Geometry check sheet. Reference: drawing and pictorial views, mm from the part's lowest x, y, z. Round coordinates to 2 decimals unless told otherwise and drop trailing zeros. Loops run counter-clockwise (first coordinate to the right, second up) from the corner with the lowest first, then second, coordinate; pieces in that order, holes last. Notation, with made-up numbers: (80, 78.25) -> (114, 78.25) arc R35 ccw to (114, 111.25) -> close; hole circle Ø9 at (78, 60). An arc over 180 degrees is marked (long way). Write item = value, one per line.
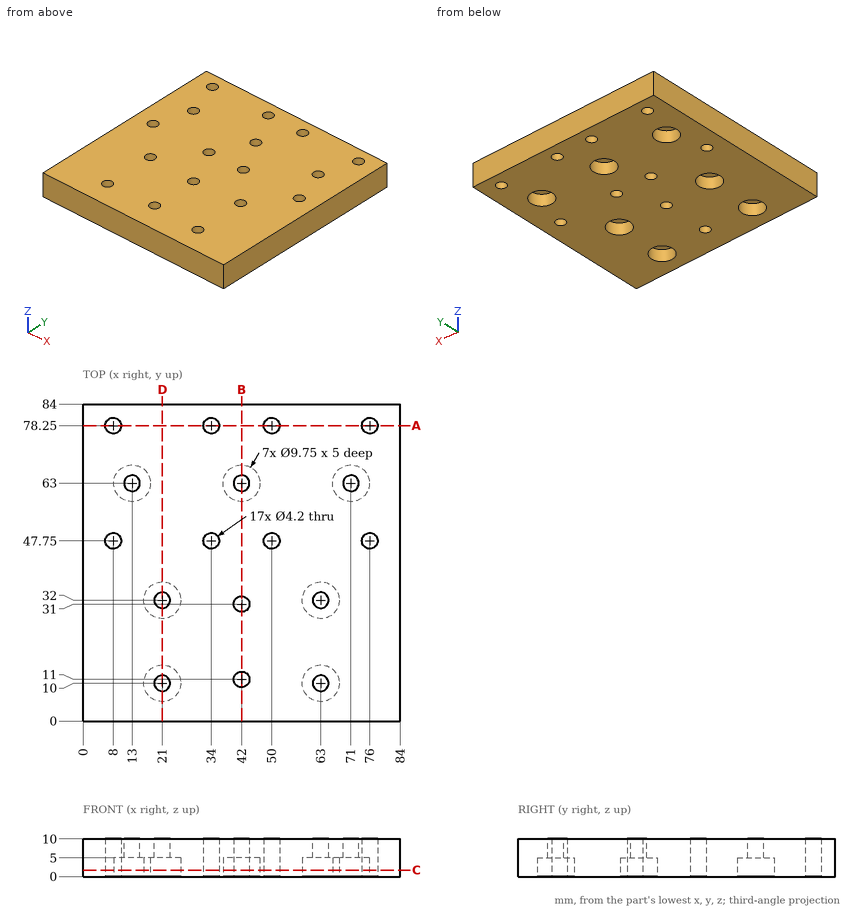
(1) Sectioned sample at A-A, the plane y = 78.25. Record the cut outline in (x, z), and give its area (3 significant figures).
Filled sheet:
outline = (0, 0) -> (5.9, 0) -> (5.9, 10) -> (0, 10) -> close; (10.1, 0) -> (31.9, 0) -> (31.9, 10) -> (10.1, 10) -> close; (36.1, 0) -> (47.9, 0) -> (47.9, 10) -> (36.1, 10) -> close; (52.1, 0) -> (73.9, 0) -> (73.9, 10) -> (52.1, 10) -> close; (78.1, 0) -> (84, 0) -> (84, 10) -> (78.1, 10) -> close
area = 672 mm2
(2) Sectioned sample at C-C, the plane z = 1.75. Count the separate pieces of the cut face and the enclosed holes in it, and give its area (3 significant figures).
Filled sheet:
separate_pieces = 1
enclosed_holes = 17
area = 6,390 mm2
(3) Sectioned sample at B-B, the plane x = 42. Record the cut outline in (y, z) (3 decimals), and give its area (3 significant figures).
Filled sheet:
outline = (0, 0) -> (8.9, 0) -> (8.9, 10) -> (0, 10) -> close; (13.1, 0) -> (28.9, 0) -> (28.9, 10) -> (13.1, 10) -> close; (33.1, 0) -> (58.125, 0) -> (58.125, 5) -> (60.9, 5) -> (60.9, 10) -> (33.1, 10) -> close; (65.1, 5) -> (67.875, 5) -> (67.875, 0) -> (84, 0) -> (84, 10) -> (65.1, 10) -> close
area = 686 mm2
(4) Go/stop test with a flat-tipped pin: pin 1 Ø5 at (x, y) = (42, 63) entering from -Z. Record where the tip stops, or that it passes through.
Filled sheet:
pin_1 = 5
(5) Material ranges on probe 1 along Y at (x, z) = (21, 6.9); probe 2 along X at (y, z) = (63, 8); probe 3 along Y at (x, z) = (76, 7.5), recorded low to high. Write a range as from..to.
Filled sheet:
probe_1 = 0..7.9, 12.1..29.9, 34.1..84
probe_2 = 0..10.9, 15.1..39.9, 44.1..68.9, 73.1..84
probe_3 = 0..45.65, 49.85..76.15, 80.35..84
(6) Sectioned sample at D-D, the plane x = 21. Record the cut outline in (y, z) (3 decimals), and give its area (4 significant figures).
Filled sheet:
outline = (0, 0) -> (5.125, 0) -> (5.125, 5) -> (7.9, 5) -> (7.9, 10) -> (0, 10) -> close; (12.1, 5) -> (14.875, 5) -> (14.875, 0) -> (27.125, 0) -> (27.125, 5) -> (29.9, 5) -> (29.9, 10) -> (12.1, 10) -> close; (34.1, 5) -> (36.875, 5) -> (36.875, 0) -> (84, 0) -> (84, 10) -> (34.1, 10) -> close
area = 700.5 mm2
